Can you work these out from the model? Positions are in its coordinate system, mm. A direction names the side the tool comes from. Give positions to 0.01 mm unless a question says otherwise; leave off trailing zeros. Order: outer loops, then holes, each group sorted by start corner. A loop starts at its lowest first (then second) coordinate and runs counter-clockwise, first axis right, second up. Notation, with made-up numbers: M -24.5,84 L 17.5,84 A19 cw 17.5,95 Z; hole C 39,61 d2. An arc over 180 degrees is marked long. Use one line per item in the form item = value. Start each with the question number.
1. I want a section at B-B, the plane z = 12.5. List the corners of the cut face in (x, y) for me, and give its area (3 significant figures).
2. I want a section at D-D, the plane x = -7. List the corners of the cut face in (y, z) for me, and give its area (3 significant figures).
3. Will these pins go through, and if not, where does the flat tip stop? P1, Ø18, axis at x = 31.5, y = 64, coming from the +Z side; P2, Ø6, axis at y = 96.5, z = 14.5, coming from the -X side; P3, Ø6, axis at x = -9, z = 13, coming from the -Y side.
4. I need wall thicknesses on L1, parallel to Y at x = 29.5, z = 6.75; L2, parallel to X at y = 27, z = 3.5; L3, parallel to Y at x = -6, z = 13.5. Which ranges of each line are inside material? Lowest first, please.
5. I want a section at C-C, the plane x = 27.5. List the corners of the cut face in (y, z) for me.
6. I want a section at A-A, the plane y = 63. List the corners of the cut face in (x, z) for me.
7. For faces 1 (the face through (32, 238, 11)), 2 (the face through (-10, 23, 10)), 3 (the face through (62, 1, 10)), which set-ups out of +Z, -Z, +X, -X, +Y, -Y let a thin tool reach every point of the face, with its end or its side?
8. We'd pull the mould along X, two halves only. Please class faces 4 (the face through (62.37, 238.296, 0.114)), 5 (the face through (62, 118, 11)), 6 (the face through (31, 122, 0)): +X half, -X half, draft (parallel to the pull), parting line (faces both ways), or undercut.
```python
from build123d import *

# Parameters (mm, degrees)
SKETCH1_W           = 64
SKETCH1_H           = 240
BOSS_EXTRUDE1_DEPTH = 19.6
FILLET1_R           = 5
CUT_EXTRUDE1_DEPTH  = 17.6
SKETCH4_W           = 19.6
SKETCH4_H           = 3
BOSS_EXTRUDE2_DEPTH = 20
FILLET2_R           = 5
CHAMFER1_SIZE       = 0.4


with BuildPart() as part:
    # Sketch1 → Boss-Extrude1 (new body)
    with BuildSketch(Plane.XY):
        with Locations((-118.769864545, 120.565422017)):
            Rectangle(SKETCH1_W, SKETCH1_H)
    extrude(amount=BOSS_EXTRUDE1_DEPTH)

    # Fillet1
    fillet1_edges = [part.edges().sort_by_distance(p)[0] for p in [
        (-86.769864545, 0.565422017, 9.8),
        (-150.769864545, 0.565422017, 9.8),
        (-150.769864545, 240.565422017, 9.8),
        (-86.769864545, 240.565422017, 9.8),
    ]]
    fillet(fillet1_edges, radius=FILLET1_R)

    # Sketch3 → Cut-Extrude1 (cut)
    with BuildSketch(Plane.XY.offset(19.6)):
        with BuildLine():
            Line((-148.769864545, 235.565422017), (-148.769864545, 5.565422017))
            ThreePointArc((-148.769864545, 5.565422017), (-147.891184888, 3.444101674), (-145.769864545, 2.565422017))
            Line((-145.769864545, 2.565422017), (-91.769864545, 2.565422017))
            ThreePointArc((-91.769864545, 2.565422017), (-89.648544201, 3.444101674), (-88.769864545, 5.565422017))
            Line((-88.769864545, 5.565422017), (-88.769864545, 235.565422017))
            ThreePointArc((-88.769864545, 235.565422017), (-89.648544201, 237.686742361), (-91.769864545, 238.565422017))
            Line((-91.769864545, 238.565422017), (-145.769864545, 238.565422017))
            ThreePointArc((-145.769864545, 238.565422017), (-147.891184888, 237.686742361), (-148.769864545, 235.565422017))
        make_face()
    extrude(amount=-CUT_EXTRUDE1_DEPTH, mode=Mode.SUBTRACT)

    # Sketch4 → Boss-Extrude2 (add)
    with BuildSketch(Plane.ZY.offset(150.769864545)):
        with Locations((9.8, 22.065422017)):
            Rectangle(SKETCH4_W, SKETCH4_H)
    extrude(amount=BOSS_EXTRUDE2_DEPTH)

    # Fillet2
    fillet2_edges = [part.edges().sort_by_distance(p)[0] for p in [
        (-170.769864545, 22.065422017, 19.6),
    ]]
    fillet(fillet2_edges, radius=FILLET2_R)


with BuildPart() as part_1:
    # Body-Move/Copy1: moved
    add(part.part.moved(Location((0, -0.56542, 0))))


with BuildPart() as part_2:
    # Body-Move/Copy2: moved
    add(part_1.part.moved(Location((150.76986, 0, 0))))

    # Chamfer1
    chamfer1_edges = [part_2.edges().sort_by_distance(p)[0] for p in [
        (31.999995455, 2.017e-06, 0),
        (63.999995455, 120.000002017, 0),
        (-4.545e-06, 129.000002017, 0),
        (31.999995455, 240.000002017, 0),
        (1.464461549, 238.535535923, 0),
        (62.535529361, 238.535535923, 0),
        (62.535529361, 1.464468112, 0),
        (1.464461549, 1.464468112, 0),
        (-4.545e-06, 12.500002017, 0),
        (-10.000004545, 23.000002017, 0),
        (-10.000004545, 20.000002017, 0),
        (-20.000004545, 21.500002017, 0),
    ]]
    chamfer(chamfer1_edges, length=CHAMFER1_SIZE)


solid = part_2.part
```
Check result:
q1.outline = M -20,20 L 0,20 L 0,5 A5 ccw 5,0 L 59,0 A5 ccw 64,5 L 64,235 A5 ccw 59,240 L 5,240 A5 ccw 0,235 L 0,23 L -20,23 Z; hole M 2,5 A3 ccw 5,2 L 59,2 A3 ccw 62,5 L 62,235 A3 ccw 59,238 L 5,238 A3 ccw 2,235 Z
q1.area = 1,250 mm2
q2.outline = M 20,0.4 L 20.4,0 L 22.6,0 L 23,0.4 L 23,19.6 L 20,19.6 Z
q2.area = 58.6 mm2
q3.P1 = 2
q3.P2 = 0
q3.P3 = 20
q4.L1 = 0 to 2, 238 to 240
q4.L2 = 0 to 2, 62 to 64
q4.L3 = 20 to 23
q5.outline = M 0,0.4 L 0.4,0 L 239.6,0 L 240,0.4 L 240,19.6 L 238,19.6 L 238,2 L 2,2 L 2,19.6 L 0,19.6 Z
q6.outline = M 0,0.4 L 0.4,0 L 63.6,0 L 64,0.4 L 64,19.6 L 62,19.6 L 62,2 L 2,2 L 2,19.6 L 0,19.6 Z
q7.face_1 = +Z
q7.face_2 = +Z, -Z, -X, +Y
q7.face_3 = +Z, -Z, +X, -Y
q8.face_4 = +X half
q8.face_5 = undercut
q8.face_6 = draft
